Here's how the part is built. I have some questions about the finished solid (model axes, mm). A direction names the side the tool comes from. Give positions to 0.01 mm unless a question says otherwise; leave off trailing zeros. Loops run counter-clockwise (first coordinate to the right, second up) from the corner with the lowest first, then second, coordinate; pieces in that order, holes last. Notation, with made-up numbers: M -8.75,68 L -3.75,68 A8 ccw -3.75,74 Z; hole C 56,-15.75 d1. An arc over 180 degrees is marked long. Answer as CSV lines item,"result". Start each with the question number.
Item 1: I want a section at A-A on z = 342.5. List the corners of the cut face in (x, y) for me.
Item 2: Will these pins go through, and if not, where does the flat tip stop? P1, Ø8, axis at x = -9, z = 112.5, coming from the -Y side; P2, Ø2, axis at x = 9, z = 294.5, coming from the -Y side; P3, Ø1, axis at x = -3, z = 61.5, coming from the -Y side; P4, Ø3, axis at x = -13, z = 151.5, coming from the +Y side.
Item 3: For faces 3 (the flat face through (6, 12.7, 207)), 4 (the cylindrical face through (-9.102, -2.72, 249.013)), 5 (the cylindrical face through (10.808, -6.67, 353.113)), 6 (the flat face through (-6, -12.7, 146)), 7 (the flat face through (-13.8, -1.5, 353.1)), which set-ups out of +Z, -Z, +X, -X, +Y, -Y let a thin tool reach every point of the face, with its end or its side?
Item 4: If I drill on line 1 along Z through (x, y) = (-5.5, -9); line 2 along Z through (x, y) = (-13.5, -1.5); line 3 along Z through (x, y) = (-3, 14), over which ranges is the centre line in solid material (lowest first)? Write a range as from..to.
Item 5: If we mould it in two halves opening along Z, with no side actions, what happens to faces 1 (the cylindrical face through (-11.18, -6.025, 207.063)), 2 (the cylindrical face through (-16.544, -9.444, 146.103))? For each: released by +Z, released by -Z, zero draft, split by the parting line, or undercut.
from build123d import *
from build123d.topology import SkipClean

# Parameters (mm, degrees)
BOSS_EXTRUDE1_DEPTH   = 3.81
BODY_MOVE_COPY2_ANGLE = 180
BOSS_EXTRUDE2_START   = -25.4
SKETCH2_R             = 9.5
BOSS_EXTRUDE2_DEPTH   = 146.05
LPATTERN1_COUNT       = 3
LPATTERN1_PITCH       = 146.05
BODY_MOVE_COPY3_ANGLE = 120
BODY_MOVE_COPY4_ANGLE = 120
BOSS_EXTRUDE3_START   = 27.94
SKETCH3_R             = 9.5
BOSS_EXTRUDE3_DEPTH   = 27.94
SKETCH4_R             = 9.5
BOSS_EXTRUDE4_DEPTH   = 15


with BuildPart() as part:
    # Sketch1 → Boss-Extrude1 (new, symmetric)
    with BuildSketch(Plane.XY):
        with BuildLine():
            Line((-5.499261314, 15.875), (-10.998522628, 6.35))
            ThreePointArc((-10.998522628, 6.35), (0, -12.7), (10.998522628, 6.35))
            Line((10.998522628, 6.35), (5.499261314, 15.875))
            ThreePointArc((5.499261314, 15.875), (0, 19.05), (-5.499261314, 15.875))
        make_face()
    extrude(amount=BOSS_EXTRUDE1_DEPTH, both=True)


with BuildPart() as body_2:
    # Body-Move_Copy1: copy of part
    add(part.part.moved(Location((0, 0, 60.96))))


with BuildPart() as body_2_1:
    # Body-Move_Copy2: moved
    add(body_2.part.rotate(Axis((0, 0, 0), (0, 0, 1)), BODY_MOVE_COPY2_ANGLE))


with BuildPart() as part_1:
    add(part.part)

    add(body_2_1.part)  # Boss-Extrude2 merges body 2
    # Sketch2 → Boss-Extrude2 (add)
    with BuildSketch(Plane.XY.offset(BOSS_EXTRUDE2_START)):
        Circle(SKETCH2_R)
    extrude(amount=BOSS_EXTRUDE2_DEPTH)


with BuildPart() as lpattern1_1:
    # LPattern1: pattern copy
    add(part_1.part.moved(Location(Vector(0, 0, 1) * (1 * LPATTERN1_PITCH))))


with BuildPart() as lpattern1_2:
    # LPattern1: pattern copy
    add(part_1.part.moved(Location(Vector(0, 0, 1) * (2 * LPATTERN1_PITCH))))


with BuildPart() as lpattern1_1_1:
    # Body-Move_Copy3: moved
    add(lpattern1_1.part.rotate(Axis((0, 0, 0), (0, 0, 1)), BODY_MOVE_COPY3_ANGLE))


with BuildPart() as lpattern1_2_1:
    # Body-Move_Copy4: moved
    add(lpattern1_2.part.rotate(Axis((0, 0, 0), (0, 0, -1)), BODY_MOVE_COPY4_ANGLE))


with BuildPart() as part_2:
    with SkipClean():  # the faces are left unmerged after this step: merging them gives an invalid solid
        add(part_1.part)

        # Sketch3 → Boss-Extrude3 (add)
        with BuildSketch(Plane(origin=(0, 0, -25.4), x_dir=(-1, 0, 0), z_dir=(0, 0, -1)).offset(BOSS_EXTRUDE3_START)):
            with Locations(Location((0, 0, 0), (0, 0, 300))):
                Circle(SKETCH3_R)
        extrude(amount=-BOSS_EXTRUDE3_DEPTH)

    # Combine1: union LPattern1_1, LPattern1_2
    add(lpattern1_1_1.part)
    add(lpattern1_2_1.part)

    # Sketch4 → Boss-Extrude4 (add)
    with SkipClean():  # the faces are left unmerged after this step: merging them gives an invalid solid
        with BuildSketch(Plane.XY.offset(412.75)):
            Circle(SKETCH4_R)
        extrude(amount=BOSS_EXTRUDE4_DEPTH)


solid = part_2.part
Result:
1,outline,"C 0,0 d19"
2,P1,"y = -8.08"
2,P2,"y = -12.7"
2,P3,"y = -18.54"
2,P4,"through"
3,face 3,"+Z, +X, -X, +Y"
3,face 4,"none"
3,face 5,"+Z"
3,face 6,"+Z, +X, -X, -Y"
3,face 7,"+Z, -X, -Y"
4,line 1,"-3.81..3.81, 57.15..64.77, 142.24..149.86, 203.2..210.82, 288.29..295.91, 349.25..356.87"
4,line 2,"142.24..149.86, 349.25..356.87"
4,line 3,"-3.81..3.81"
5,face 1,"undercut"
5,face 2,"zero draft"
